Check sheet for the drawn part. Datum: minimum x, y, z corner. Units: mm. A direction names the side the tool comes from. Round coordinates to 2 decimals unless told otherwise and drop trailing zeros. Order: outer loops, then holes, each group sorted by start corner. A loop starts at its lowest first (then second) coordinate and runs counter-clockwise, first axis right, second up. Notation, with made-up numbers: M 28.5,3.25 L 45.5,3.25 A12 cw 45.5,20.25 Z; hole C -30.75,74.25 d6. An arc over 180 degrees is marked long. Use one line per item in the form item = value. Start each with the question number.
Item 1: Go/stop test with flat-tipped pins: pin 1 Ø1.2 at (y, z) = (30, 2.5) entering from +X; pin 2 Ø1.5 at (y, z) = (21, 3.5) entering from -X; pin 3 Ø4 at (x, y) = (64, 29) entering from -Z; pin 4 Ø8 at (x, y) = (20, 36) entering from -Z. Record where each tip stops, or that it passes through.
Item 2: Tool access check on the marked faces 1, 2, 3, 4 and 5. Record the directions out of +Z, -Z, +X, -X, +Y, -Y that give a thin tool (end or side, any length) a straight path to the whole face; none if there is none.
Item 3: Thickness scan on probe 1 along Y at (x, z) = (41.5, 3.25); probe 2 along Y at (x, z) = (36, 4.75); probe 3 along X at (y, z) = (28, 8.25). Record the ranges inside material, lowest first. Write a range as [from, to].
Item 4: Cross-section at A-A on x = 34.5. Enter the section's corners in (y, z), then the cut area to 3 significant figures.
Item 5: Cross-section at C-C on y = 46.5. Enter the section's corners in (x, z).
Item 6: Cross-section at B-B on z = 7.5. Enter the section's corners in (x, y), then the cut area to 3 significant figures.
Item 7: Cross-section at D-D on x = 60.5. Enter the section's corners in (y, z), then the cut area to 3 significant figures.
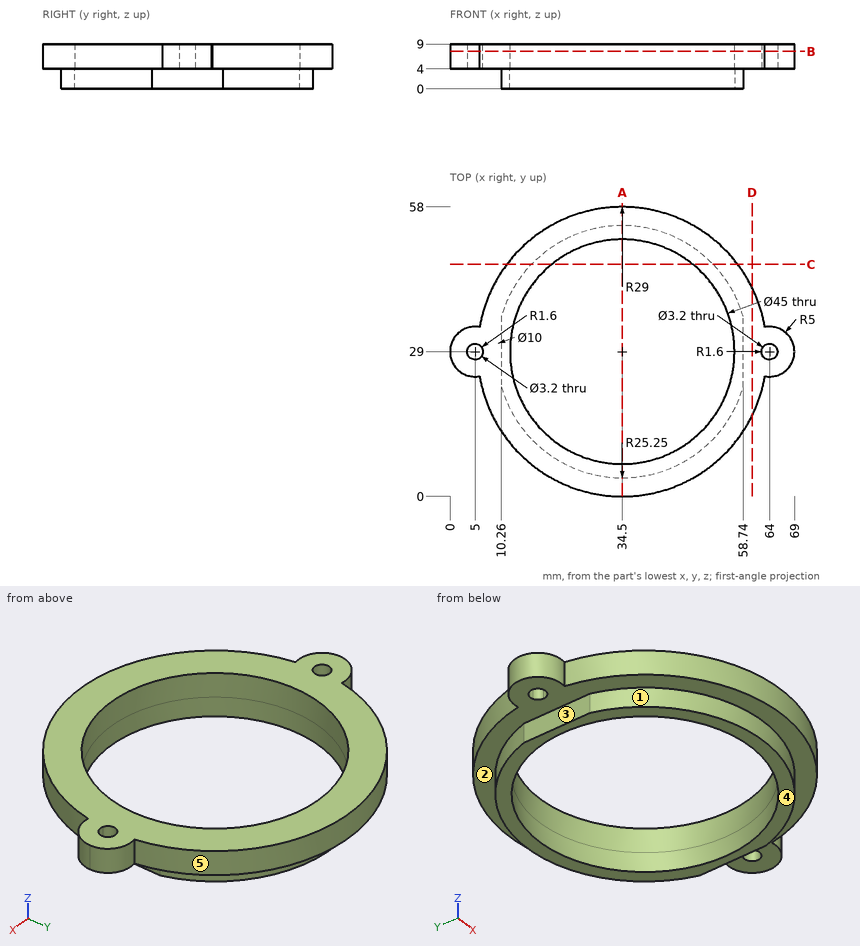
Output values:
q1.pin_1 = 58.74
q1.pin_2 = 6.47
q1.pin_3 = 4
q1.pin_4 = through
q2.face_1 = -Z, -Y
q2.face_2 = -Z
q2.face_3 = -Z, -X, +Y, -Y
q2.face_4 = -Z, +X, -X, +Y, -Y
q2.face_5 = +Z, -Z, +Y
q3.probe_1 = [4.74, 7.62], [50.38, 53.26]
q3.probe_2 = [0.04, 6.55], [51.45, 57.96]
q3.probe_3 = [0.1, 3.75], [6.25, 12.02], [56.98, 62.75], [65.25, 68.9]
q4.outline = M 0,4 L 3.75,4 L 3.75,0 L 6.5,0 L 6.5,9 L 0,9 Z; M 51.5,0 L 54.25,0 L 54.25,4 L 58,4 L 58,9 L 51.5,9 Z
q4.area = 87.0 mm2
q5.outline = M 11.38,4 L 16.3,4 L 16.3,0 L 20.36,0 L 20.36,9 L 11.38,9 Z; M 48.64,0 L 52.7,0 L 52.7,4 L 57.62,4 L 57.62,9 L 48.64,9 Z
q6.outline = M 5.92,24.09 A29 ccw 63.08,24.09 A5 ccw long 63.08,33.91 A29 ccw 5.92,33.91 A5 ccw long Z; hole C 5,29 d3.2; hole C 34.5,29 d45; hole C 64,29 d3.2
q6.area = 1,130 mm2
q7.outline = M 16.15,4 L 41.85,4 L 41.85,9 L 16.15,9 Z
q7.area = 128 mm2
